Autodesk Fusion 360 part; units mm, degrees
sketch "Sketch1" plane through (0, 0, 0) normal (0, 1, 0) x (1, 0, 0)
  line L0 (-25, 0) -> (-25, 5)
  line L1 (-25, 5) -> (-25, 19)
  line L2 (-25, 19) -> (-21, 19)
  line L3 (-21, 19) -> (-21, 5)
  line L4 (-21, 5) -> (-11, 5)
  line L5 (-11, 5) -> (-11, 19)
  line L6 (-11, 19) -> (-7, 19)
  line L7 (-7, 19) -> (-7, 5)
  line L8 (-7, 5) -> (-2.5, 5)
  line L9 (-2.5, 5) -> (7.5, 5)
  line L10 (7.5, 5) -> (7.5, 0)
  line L11 (-25, 0) -> (-2.5, 0)
  line L12 (7.5, 0) -> (7.5, -5)
  line L13 (-7.4852, -82.9997) -> (-2.5, -83)
  spline S0 degree 5 poles (-7.4852, -82.9997) (-7.0499, -82.9476) (-6.1946, -82.8346) (-4.9577, -82.6382) (-3.4023, -82.3219) (-1.6257, -81.829) (-0.0341, -81.2286) (1.3528, -80.509) (2.5178, -79.6605) (3.4572, -78.6808) (4.1826, -77.5767) (4.6031, -76.6004) (4.8339, -75.819) (4.9508, -75.2766) (5, -75) knots 0 0 0 0 0 0 0.1 0.2 0.3 0.4 0.5 0.6 0.7 0.8 0.9 1 1 1 1 1 1
  line L14 (-2.5, 0) -> (5, -75)
  line L15 (5, -75) -> (7.5, -75)
  line L16 (7.5, -5) -> (7.5, -75)
  spline S1 degree 5 poles (-2.5, -83) (-2.0851, -82.9482) (-1.2732, -82.8357) (-0.1087, -82.64) (1.3356, -82.3244) (2.947, -81.8324) (4.3443, -81.2324) (5.5048, -80.5132) (6.4084, -79.6647) (7.0507, -78.6846) (7.4451, -77.5796) (7.5755, -76.6023) (7.5752, -75.8201) (7.5322, -75.277) (7.5, -75) knots 0 0 0 0 0 0 0.1 0.2 0.3 0.4 0.5 0.6 0.7 0.8 0.9 1 1 1 1 1 1
  point P0 (2, -80)
  point P1 (6, -80)
extrude "Extrude1" add sketch "Sketch1" along normal blind 30
sketch "Sketch2" plane through (-25, 0, 0) normal (-1, 0, 0) x (0, 0, 1)
  line L0 (-19, 0) -> (0, 0)
  line L1 (0, 0) -> (0, 30)
  line L2 (0, 30) -> (-19, 30)
  line L3 (-19, 30) -> (-19, 0)
  line L4 (0, 30) -> (-9, 30)
  line L5 (-9, 0) -> (0, 0)
  line L6 (0, 0) -> (0, 30)
  line L7 (-9, 30) -> (-19, 30)
  line L8 (-19, 30) -> (-19, 21)
  line L9 (-19, 21) -> (-9, 21)
  line L10 (-9, 0) -> (-19, 0)
  line L11 (-19, 0) -> (-19, 9)
  line L12 (-19, 9) -> (-9, 9)
  line L13 (-9, 21) -> (-19, 21)
  line L14 (-19, 21) -> (-19, 9)
  line L15 (-19, 9) -> (-9, 9)
  line L16 (-9, 9) -> (-9, 21)
extrude "Extrude2" cut sketch "Sketch2" against normal blind 4 contours L3 L9 L12 L13 L14 L15 L16
sketch "Sketch3" plane through (-7, 0, 0) normal (1, 0, 0) x (0, 0, -1)
  line L0 (5, 0) -> (19, 0)
  line L1 (19, 0) -> (19, 30)
  line L2 (19, 30) -> (5, 30)
  line L3 (5, 30) -> (5, 0)
  line L4 (5, 0) -> (19, 0)
  line L5 (19, 0) -> (19, 6)
  line L6 (19, 6) -> (5, 6)
  line L7 (5, 6) -> (5, 0)
  line L8 (5, 30) -> (19, 30)
  line L9 (19, 30) -> (19, 24)
  line L10 (19, 24) -> (5, 24)
  line L11 (5, 24) -> (5, 30)
  dimension "d29" = 6
  dimension "d30" = 6
extrude "Extrude3" cut sketch "Sketch3" against normal blind 4 contours L1 L3 L6 L10
Model file for the job. Use its own axes, mm. A direction names the side the tool comes from. Give positions to 0.01 mm unless a question says otherwise; leave off trailing zeros. Order: outer loops, then holes, each group sorted by start corner. A loop starts at its lowest first (then second) coordinate and runs counter-clockwise, first axis right, second up. Notation, with made-up numbers: (-4, -38) - (16, -38) arc R17 cw to (16, -8) - close; hole circle Ø3 at (88, 82). An arc over 180 degrees is marked (long way). Write item = value, one per line. Start each with the question number.
1. Cut at A-A, the plane x = -10. List the corners of the cut face in (y, z), and give its area (3 significant figures).
2. Drop flat-ended pins along their axis: P1, Ø1.2, axis at x = -22.5, y = 14, coming from the -Z side; P2, Ø6.5, axis at y = 2, z = -15.5, coming from the +X side; P3, Ø10, axis at x = -18.5, y = 13, coming from the +Z side; P4, Ø7, axis at y = 17, z = -14, coming from the +X side. Give the stop position or say it passes through.
3. Cut at B-B, the plane z = 20. List the corners of the cut face in (x, y), and give its area (3 significant figures).
4. Cut at C-C, the plane z = 53.5. List the corners of the cut face in (x, y), and give its area (4 significant figures).
5. Probe line 1 along Y through (x, z) = (-9, -10); line 2 along X through (y, z) = (25, -15); line 3 along Z through (x, y) = (-18.5, 4.5). List the from-to ranges inside material, lowest first.
6. Two-plate mould, pull along X, no slides. Class faces 5 (the flat face through (-11, 27, -12)), 6 (the flat face through (7.5, 15, 34)), 7 (the flat face through (-9, 3, -19)): pulls with the +X half, pulls with the -X half, needs draft (parallel to the pull), parting line crosses it, or undercut.
7. Which spindle directions (+Z, -Z, +X, -X, +Y, -Y) get a long thin tool onto all of the face, cutting with end or side? Do faces 1 (the flat face through (1.2, 14.8, 37)), 2 (the flat face through (-9, 6, -12)), 3 (the flat face through (-23, 21, -14)), 4 (the flat face through (-7, 27, -12)). Say none if no direction does.
Taken from the geometry:
q1.outline = (0, -19) - (6, -19) - (6, -5) - (24, -5) - (24, -19) - (30, -19) - (30, 0) - (0, 0) - close
q1.area = 318 mm²
q2.P1 = -9
q2.P2 = -7
q2.P3 = 0
q2.P4 = through
q3.outline = (-0.5, 0) - (7.5, 0) - (7.5, 30) - (-0.5, 30) - close
q3.area = 240 mm²
q4.outline = (2.85, 0) - (7.5, 0) - (7.5, 30) - (2.85, 30) - close
q4.area = 139.5 mm²
q5.line_1 = 0 to 6, 24 to 30
q5.line_2 = -25 to -21, -11 to -7
q5.line_3 = -5 to 0
q6.face_5 = undercut
q6.face_6 = pulls with the +X half
q6.face_7 = needs draft
q7.face_1 = -X, +Y, -Y
q7.face_2 = -Z, +X
q7.face_3 = -Z, +X, -X
q7.face_4 = -Z, +X, +Y, -Y
